from build123d import *

# Parameters (mm, degrees)
SKETCH1_W           = 96
SKETCH1_H           = 160
BOSS_EXTRUDE1_DEPTH = 100
SKETCH2_R           = 12.5
CUT_EXTRUDE1_DEPTH  = 195.689496378
CHAMFER1_SIZE       = 10


with BuildPart() as part:
    # Sketch1 → Boss-Extrude1 (new body)
    with BuildSketch(Plane.XY):
        with Locations((0, 80)):
            Rectangle(SKETCH1_W, SKETCH1_H)
    extrude(amount=BOSS_EXTRUDE1_DEPTH)

    # Sketch2 → Cut-Extrude1 (cut, through all)
    with BuildSketch(Plane.XY.offset(100)):
        with Locations((0, 125)):
            Circle(SKETCH2_R)
    extrude(amount=-CUT_EXTRUDE1_DEPTH, mode=Mode.SUBTRACT)

    # Chamfer1
    chamfer1_edges = [part.edges().sort_by_distance(p)[0] for p in [
        (-48, 160, 50),
        (48, 160, 50),
    ]]
    chamfer(chamfer1_edges, length=CHAMFER1_SIZE)


solid = part.part
Source: CAD feature listing. Evaluate the final solid. Frame: model axes, mm. Give positions to 0.01 mm unless a question says otherwise; leave off trailing zeros. Write each loop counter-clockwise with the first axis right and the second up, starting at its lowest first coordinate (ties: lowest second). Pieces come first, ordered by that corner, then holes. Notation, with made-up numbers: (-39.75, 70) -> (-24.75, 70) arc R24 cw to (-24.75, 99) -> close; hole circle Ø1 at (11.5, 48). An arc over 180 degrees is marked (long way). Write item = value, one per line.
Q1. Cut plane C-C on z = 72. Return loops of the section in (x, y), then the cut area to 3 significant figures.
Here are the results:
outline = (-48, 0) -> (48, 0) -> (48, 150) -> (38, 160) -> (-38, 160) -> (-48, 150) -> close; hole circle Ø25 at (0, 125)
area = 14,800 mm²
Q2. Mould query, pull axis X, two halves, no side actions, for faces 1 (the face through (48, 74, 49)), 2 (the face through (-1, 160, 49)), 3 (the face through (-1.627, 137.394, 50.7)), 4 (the face through (-43, 155, 49)). Classes: +X half, -X half, draft (parallel to the pull), parting line (faces both ways), or undercut.
Here are the results:
face_1 = +X half
face_2 = draft
face_3 = undercut
face_4 = -X half
Q3. Cut plane B-B on y = 116.5. Return loops of the section in (x, z).
Here are the results:
outline = (-48, 0) -> (-9.17, 0) -> (-9.17, 100) -> (-48, 100) -> close; (9.17, 0) -> (48, 0) -> (48, 100) -> (9.17, 100) -> close
Q4. Line query: line 1 (Y direction, x = 0, z = 77); line 2 (Y direction, x = -4, z = 87.5); line 3 (X direction, y = 131, z = 40.5). Output: solid intervals per line, ascending. Write a range as from..to.
Here are the results:
line_1 = 0..112.5, 137.5..160
line_2 = 0..113.16, 136.84..160
line_3 = -48..-10.97, 10.97..48
Q5. Cut plane A-A on x = 0. Return loops of the section in (y, z).
Here are the results:
outline = (0, 0) -> (112.5, 0) -> (112.5, 100) -> (0, 100) -> close; (137.5, 0) -> (160, 0) -> (160, 100) -> (137.5, 100) -> close
